Could you check a few things on this drawing? It's one solid part, dimensions in mm from its lowest x, y, z. A direction names the side the tool comes from. Give positions to 0.01 mm unless a question says otherwise; leave off trailing zeros. Order: outer loops, then holes, each group sorted by start corner. A loop starts at its lowest first (then second) coordinate and runs counter-clockwise, first axis right, second up. Notation, with made-up numbers: M 22.25,37.5 L 55.25,37.5 A27 ccw 55.25,70.5 Z; hole C -21,-15.75 d6. An arc over 180 degrees is marked long. Use CSV: the item, a comma, the result in double quotes. Start each with the question number.
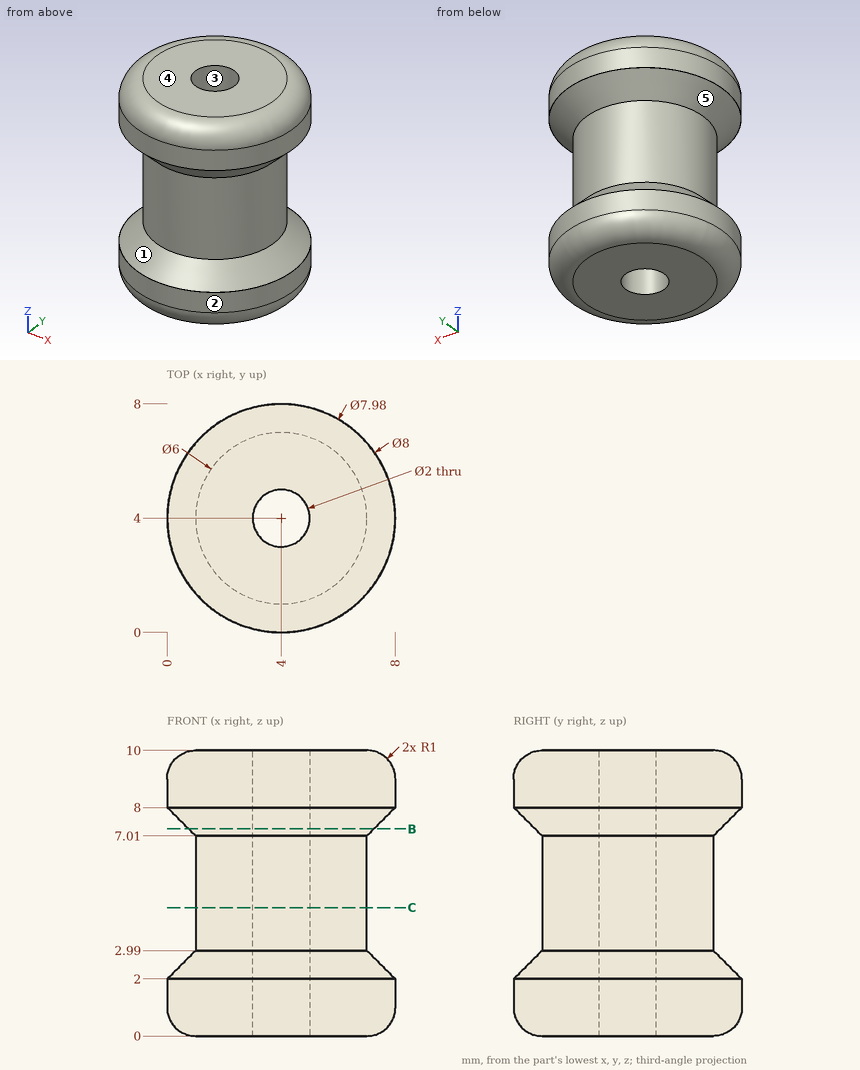
Q1. We'd pull the mould along X, two halves only. Please class the marked faces 3, 4 and 5: pulls with the +X half, pulls with the -X half, needs draft (parallel to the pull), parting line crosses it, or undercut.
Q2. For P1, Ø1, axis at x = 2.5, z = 1, coming from the +Y side; P2, Ø4, axis at x = 6, z = 6, coming from the -Y side; P3, Ø4, axis at y = 2, z = 6.5, coming from the +X side, each with a flat end and sliding along its axis, tell me the tip position at first contact or that it passes through.
Q3. Imagine slicing it at B-B, the plane z = 7.25. Please give me the cut outline in (x, y), then the cut area to 3 significant figures.
Q4. I need wall thicknesses on line 1 (Y direction, x = 4, z = 3.75); line 2 (Z direction, x = 1.25, y = 1.5); line 3 (Z direction, x = 1, y = 4.5). Which ranges of each line are inside material? Lowest first, please. Write a range as [from, to].
Q5. Imagine slicing it at C-C, the plane z = 4.5. Please give me the cut outline in (x, y), then the cut area to 3 significant figures.
Q6. For the marked faces 1 and 2, which set-ups out of +Z, -Z, +X, -X, +Y, -Y let a thin tool reach every point of the face, with its end or its side?
Reply:
1,face 3,"undercut"
1,face 4,"needs draft"
1,face 5,"parting line crosses it"
2,P1,"stops at y = 7.87"
2,P2,"stops at y = 0.36"
2,P3,"stops at x = 7.94"
3,outline,"C 4,4 d6.48; hole C 4,4 d2"
3,area,"29.8 mm^2"
4,line 1,"y = [1, 3], [5, 7]"
4,line 2,"z = [0.3, 2.27], [7.73, 9.7]"
4,line 3,"z = [0, 2.95], [7.05, 10]"
5,outline,"C 4,4 d6; hole C 4,4 d2"
5,area,"25.1 mm^2"
6,face 1,"none"
6,face 2,"+Z, -Z"
